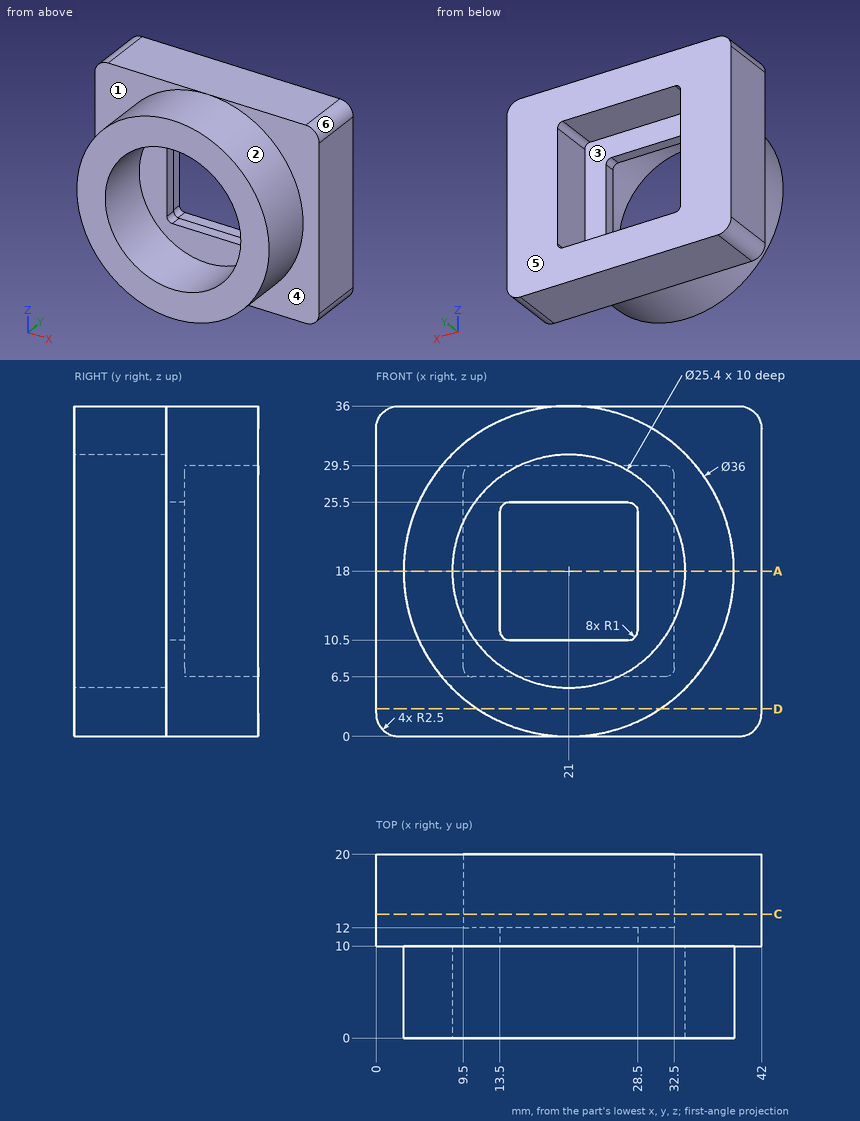
Verification items for this drawing (mm, ordinates from the low corner). A direction names the side the tool comes from. Give positions to 0.01 mm unless a question says otherwise; leave off trailing zeros. Loops run counter-clockwise (first coordinate to the right, second up) from the corner with the lowest first, then second, coordinate; pieces in that order, holes last. Notation, with made-up numbers: M 56,14 L 100,14 A9 ccw 100,31 Z; hole C 44.5,2.25 d4. An arc over 180 degrees is marked long. Return JSON: item names as keys, results as strings. Group by question number.
1. Thickness scan on L1, parallel to X at y = 13.5, z = 9.5; L2, parallel to X at y = 10.25, z = 19.5; L3, parallel to Z at x = 21, y = 2.75. Record the ranges inside material, lowest first.
2. Tool access check on the marked faces 1, 2 and 3. Record the directions out of +Z, -Z, +X, -X, +Y, -Y that give a thin tool (end or side, any length) a straight path to the whole face; none if there is none.
3. Mould release check, pull along Y, two halves, no side actions. Record for the marked faces 4, 5 and 6: released by +Y, released by -Y, zero draft, split by the parting line, or undercut.
4. Go/stop test with flat-tipped pins: pin 1 (2 mm diameter, centred on x = 24.5, y = 3, fed in from +Z); pin 2 (11.5 mm diameter, centred on x = 16, z = 21, fed in from +Y); pin 3 (3 mm diameter, centred on y = 2.5, z = 29.5, fed in from +X). Record where each tip stops, or that it passes through.
5. Cross-section at D-D on z = 3. Record the boundary of the cut face in (x, y).
6. Cross-section at C-C on y = 13.5. Record the boundary of the cut face in (x, z).
7. Cross-section at A-A on z = 18. Record the boundary of the cut face in (x, y), plus the area to 3 significant figures.
Return value:
{
 "1": {"L1": "0 to 9.5, 32.5 to 42", "L2": "0 to 13.5, 28.5 to 42", "L3": "0 to 5.3, 30.7 to 36"},
 "2": {"face 1": "-X, -Y", "face 2": "-Y", "face 3": "+Y"},
 "3": {"face 4": "released by -Y", "face 5": "released by +Y", "face 6": "zero draft"},
 "4": {"pin 1": "z = 35.83", "pin 2": "y = 12", "pin 3": "x = 35.97"},
 "5": {"outline": "M 0,10 L 11.05,10 L 11.05,0 L 30.95,0 L 30.95,10 L 42,10 L 42,20 L 0,20 Z"},
 "6": {"outline": "M 0,2.5 A2.5 ccw 2.5,0 L 39.5,0 A2.5 ccw 42,2.5 L 42,33.5 A2.5 ccw 39.5,36 L 2.5,36 A2.5 ccw 0,33.5 Z; hole M 9.5,7.5 A1 ccw 10.5,6.5 L 31.5,6.5 A1 ccw 32.5,7.5 L 32.5,28.5 A1 ccw 31.5,29.5 L 10.5,29.5 A1 ccw 9.5,28.5 Z"},
 "7": {"outline": "M 0,10 L 3,10 L 3,0 L 8.3,0 L 8.3,10 L 13.5,10 L 13.5,12 L 9.5,12 L 9.5,20 L 0,20 Z; M 28.5,10 L 33.7,10 L 33.7,0 L 39,0 L 39,10 L 42,10 L 42,20 L 32.5,20 L 32.5,12 L 28.5,12 Z", "area": "312 mm^2"}
}
